```python
from build123d import *

# Parameters (mm, degrees)
SKETCH3_R           = 1.6
BOSS_EXTRUDE1_DEPTH = 5
SKETCH4_W           = 3
SKETCH4_H           = 23.5
BOSS_EXTRUDE2_DEPTH = 6
SKETCH5_R           = 1.6
CUT_EXTRUDE1_DEPTH  = 136
SKETCH6_W           = 4.7
SKETCH6_H           = 12
SKETCH6_R           = 1.6
BOSS_EXTRUDE3_DEPTH = 28.65
SKETCH8_W           = 6
SKETCH8_H           = 2.7
CUT_EXTRUDE3_DEPTH  = 98.45
FILLET1_R           = 2
CHAMFER1_SIZE       = 2
SKETCH9_R           = 1.333333333
CUT_EXTRUDE4_DEPTH  = 25
FILLET2_R           = 2


with BuildPart() as part:
    # Sketch3 → Boss-Extrude1 (new body)
    with BuildSketch(Plane(origin=(0, 0, 0), x_dir=(1, 0, 0), z_dir=(0, 1, 0))):
        Polygon((39.9, 17.5), (-95.1, 17.5), (-95.1, -6), (-80.560784084, -6), (-80.560784084, -9.5), (-58.560784084, -9.5), (-58.560784084, -6), (-35.1, -6), (-35.1, -24), (-20.1, -24), (-20.1, -6), (39.9, -6), align=None)
        with Locations((-63.560784084, -6)):
            Circle(SKETCH3_R, mode=Mode.SUBTRACT)
        with Locations((-75.560784084, -6)):
            Circle(SKETCH3_R, mode=Mode.SUBTRACT)
        with Locations((8.4, 5.75)):
            Circle(SKETCH3_R, mode=Mode.SUBTRACT)
        with Locations((28.4, 5.75)):
            Circle(SKETCH3_R, mode=Mode.SUBTRACT)
        with Locations((-27.6, -9)):
            Circle(SKETCH3_R, mode=Mode.SUBTRACT)
        with Locations((-27.6, -21)):
            Circle(SKETCH3_R, mode=Mode.SUBTRACT)
    extrude(amount=BOSS_EXTRUDE1_DEPTH)

    # Sketch4 → Boss-Extrude2 (add)
    with BuildSketch(Plane.XZ):
        with Locations((38.4, -5.75)):
            Rectangle(SKETCH4_W, SKETCH4_H)
        with Locations((28.1, -5.75)):
            Rectangle(SKETCH4_W, SKETCH4_H)
        with Locations((-93.6, -5.75)):
            Rectangle(SKETCH4_W, SKETCH4_H)
        with Locations((-83.3, -5.75)):
            Rectangle(SKETCH4_W, SKETCH4_H)
    extrude(amount=BOSS_EXTRUDE2_DEPTH)

    # Sketch5 → Cut-Extrude1 (cut, through all)
    with BuildSketch(Plane(origin=(39.9, 0, 0), x_dir=(0, 0, -1), z_dir=(1, 0, 0))):
        with Locations((11.5, -3.55)):
            Circle(SKETCH5_R)
    extrude(amount=-CUT_EXTRUDE1_DEPTH, mode=Mode.SUBTRACT)

    # Sketch6 → Boss-Extrude3 (add)
    with BuildSketch(Plane.XZ):
        with Locations((-55.2, 0)):
            Rectangle(SKETCH6_W, SKETCH6_H)
        with Locations((-55.2, 0)):
            Circle(SKETCH6_R, mode=Mode.SUBTRACT)
        Rectangle(SKETCH6_W, SKETCH6_H)
        Circle(SKETCH6_R, mode=Mode.SUBTRACT)
    extrude(amount=BOSS_EXTRUDE3_DEPTH)

    # Sketch8 → Cut-Extrude3 (cut, through all)
    with BuildSketch(Plane.ZY.offset(57.55)):
        with Locations((0, -16.65)):
            Rectangle(SKETCH8_W, SKETCH8_H)
    extrude(amount=-CUT_EXTRUDE3_DEPTH, mode=Mode.SUBTRACT)

    # Fillet1
    fillet1_edges = [part.edges().sort_by_distance(p)[0] for p in [
        (39.9, 5, -5.75),
        (-95.1, 5, -5.75),
    ]]
    fillet(fillet1_edges, radius=FILLET1_R)

    # Chamfer1
    chamfer1_edges = [part.edges().sort_by_distance(p)[0] for p in [
        (-52.85, -14.325, -6),
        (-2.35, -14.325, -6),
    ]]
    chamfer(chamfer1_edges, length=CHAMFER1_SIZE)

    # Sketch9 → Cut-Extrude4 (cut)
    with BuildSketch(Plane(origin=(0, 0, 0), x_dir=(1, 0, 0), z_dir=(0, 1, 0))):
        with Locations((-3.1, 9.5)):
            Circle(SKETCH9_R)
        with Locations((-52.1, 9.5)):
            Circle(SKETCH9_R)
    extrude(amount=CUT_EXTRUDE4_DEPTH, mode=Mode.SUBTRACT)

    # Fillet2
    fillet2_edges = [part.edges().sort_by_distance(p)[0] for p in [
        (-58.560784084, 2.5, 9.5),
        (-80.560784084, 2.5, 9.5),
        (-20.1, 2.5, 24),
        (-35.1, 2.5, 24),
    ]]
    fillet(fillet2_edges, radius=FILLET2_R)


solid = part.part
```
Could you check a few things on this model? Use its own coordinates, in mm. A direction names the side the tool comes from. Coordinates: 2 decimals unless noted, no trailing zeros. Write each loop counter-clockwise with the first axis right and the second up, starting at its lowest first coordinate (ties: lowest second). Pieces come first, ordered by that corner, then holes. Notation, with made-up numbers: M 50,50.5 L 87,50.5 A15 cw 87,64.5 Z; hole C -22,45 d10. An arc over 180 degrees is marked long. Answer as CSV lines item,"result". Start each with the question number.
1) Please list where these lines run through material, in increasing order: line 1 (Z direction, x = -27, y = 3); line 2 (Z direction, x = 0, y = -20.5); line 3 (Y direction, x = -87, z = -5.5). Write a range as from..to.
2) For P1, Ø2.5, axis at x = 28.4, z = -5.75, coming from the -Y side; P2, Ø5, axis at y = -20, z = 0, coming from the -X side; P3, Ø1.4, axis at x = -56, y = -17.5, coming from the +Z side; P4, Ø4, axis at y = -3.55, z = -11.5, coming from the +X side, each with a flat end and sliding along its axis, tell me the tip position at first contact or that it passes through.
3) I want a section at C-C, the plane x = 5. Please give me the cut outline in (y, z), and give its area (4 significant figures).
4) I want a section at B-B, the plane x = 28.4. Please give me the cut outline in (y, z), and give its area (3 significant figures).
5) I want a section at A-A, the plane y = -12.5. Please give me the cut outline in (x, z), and give its area (3 significant figures).
6) For faces 4 (the flat face through (28, 0, -6)), 5 (the flat face through (38, -6, -6)), 6 (the flat face through (-2, -15.3, 0)), 7 (the cylindrical face through (-1.27, -7.54, -0.97)), which set-ups out of +Z, -Z, +X, -X, +Y, -Y let a thin tool reach every point of the face, with its end or its side?
7) We'd pull the mould along X, two halves only. Please class faces 1 (the flat face through (-55, -17, 3)), 2 (the flat face through (-95.1, -2, -6)), 3 (the flat face through (1, -14, -6)): +X half, -X half, draft (parallel to the pull), parting line (faces both ways), or undercut.
Data:
1,line 1,"z = -17.5..7.52, 10.48..19.52, 22.48..24"
1,line 2,"z = -6..-1.6, 1.6..6"
1,line 3,"y = 0..5"
2,P1,"stops at y = -6"
2,P2,"stops at x = -57.55"
2,P3,"stops at z = 6"
2,P4,"stops at x = 39.9"
3,outline,"M 0,-17.5 L 5,-17.5 L 5,6 L 0,6 Z"
3,area,"117.5 mm^2"
4,outline,"M -6,-17.5 L 5,-17.5 L 5,-7.35 L 0,-7.35 L 0,-4.15 L 5,-4.15 L 5,6 L -6,6 Z; hole C -3.55,-11.5 d3.2"
4,area,"234 mm^2"
5,outline,"M -57.55,-6 L -54.85,-6 L -52.85,-4 L -52.85,6 L -57.55,6 Z; M -2.35,-4 L -0.35,-6 L 2.35,-6 L 2.35,6 L -2.35,6 Z; hole C -55.2,0 d3.2; hole C 0,0 d3.2"
5,area,"92.7 mm^2"
6,face 4,"+Y"
6,face 5,"+Z, -Z, +X, -Y"
6,face 6,"+X, -X"
6,face 7,"-Y"
7,face 1,"draft"
7,face 2,"-X half"
7,face 3,"undercut"
